Could you check a few things on this model? Use its own coordinates, in mm. Face numbers are marked on the shaded views. A direction names the side the tool comes from. Coordinates: 2 decimals unless noted, no trailing zeros. Loops run counter-clockwise (first coordinate to the right, second up) from the corner with the lowest first, then second, coordinate; pieces in that order, holes last. Notation, with made-up numbers: (-4, 42) - (54, 42) arc R14 cw to (54, 46) - close; hole circle Ø9 at (75, 46.5). An arc over 180 degrees is marked (long way). Use CSV: the item, a comma, the result in double quotes.
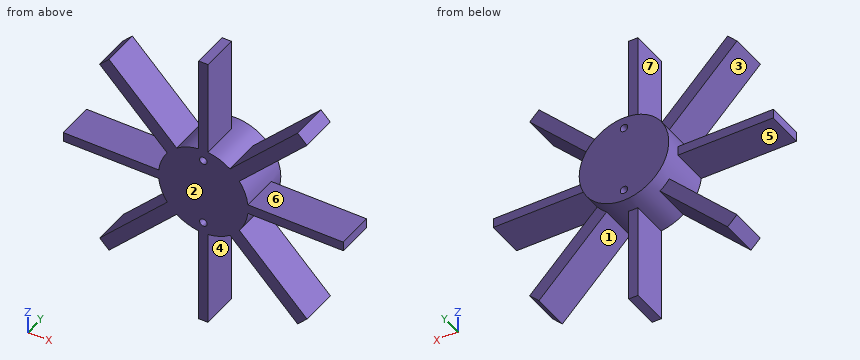
Autodesk Inventor part; units mm, degrees
ref_plane "YZ Plane" through (0, 0, 0) normal (1, 0, 0) x (0, 1, 0)
ref_plane "XZ Plane" through (0, 0, 0) normal (0, 1, 0) x (-1, 0, 0)
ref_plane "XY Plane" through (0, 0, 0) normal (0, 0, 1) x (1, 0, 0)
sketch "Sketch2" plane through (0, 0, 0) normal (0, 1, 0) x (-1, 0, 0)
  circle A0 centre (0, 0) radius 12
  line L0 (-1.25, 37.5) -> (-1.25, -37.5)
  line L1 (-1.25, -37.5) -> (1.25, -37.5)
  line L2 (1.25, -37.5) -> (1.25, 37.5)
  line L3 (1.25, 37.5) -> (-1.25, 37.5)
  line L4 (-1.25, 37.5) -> (1.25, -37.5) construction
  line L5 (-1.25, -37.5) -> (1.25, 37.5) construction
  line L6 (-37.5, -1.25) -> (37.5, -1.25)
  line L7 (37.5, -1.25) -> (37.5, 1.25)
  line L8 (37.5, 1.25) -> (-37.5, 1.25)
  line L9 (-37.5, 1.25) -> (-37.5, -1.25)
  line L10 (-37.5, -1.25) -> (37.5, 1.25) construction
  line L11 (37.5, -1.25) -> (-37.5, 1.25) construction
  line L12 (1.25, 1.25) -> (-1.25, -1.25)
  line L13 (-1.25, -1.25) -> (25.2665, -27.7665)
  line L14 (25.2665, -27.7665) -> (27.7665, -25.2665)
  line L15 (27.7665, -25.2665) -> (1.25, 1.25)
  line L16 (1.25, 1.25) -> (-1.25, -1.25)
  line L17 (-1.25, -1.25) -> (-27.7665, 25.2665)
  line L18 (-27.7665, 25.2665) -> (-25.2665, 27.7665)
  line L19 (-25.2665, 27.7665) -> (1.25, 1.25)
  line L20 (-1.25, 1.25) -> (1.25, -1.25)
  line L21 (1.25, -1.25) -> (-25.2665, -27.7665)
  line L22 (-25.2665, -27.7665) -> (-27.7665, -25.2665)
  line L23 (-27.7665, -25.2665) -> (-1.25, 1.25)
  line L24 (-1.25, 1.25) -> (1.25, -1.25)
  line L25 (1.25, -1.25) -> (27.7665, 25.2665)
  line L26 (27.7665, 25.2665) -> (25.2665, 27.7665)
  line L27 (25.2665, 27.7665) -> (-1.25, 1.25)
  point P0 (7.1427, -9.6427)
  point P1 (9.6427, -7.1427)
  point P2 (11.9347, -1.25)
  point P3 (11.9347, 1.25)
  point P4 (9.6427, 7.1427)
  point P5 (7.1427, 9.6427)
  point P6 (1.25, 11.9347)
  point P7 (-1.25, 11.9347)
  point P8 (-7.1427, 9.6427)
  point P9 (-9.6427, 7.1427)
  point P10 (-11.9347, 1.25)
  point P11 (-11.9347, -1.25)
  point P12 (-9.6427, -7.1427)
  point P13 (-7.1427, -9.6427)
  point P14 (-1.25, -11.9347)
  point P15 (1.25, -11.9347)
  dimension "d0" = 24
  dimension "d1" = 75
  dimension "d2" = 2.5
  dimension "d3" = 75
  dimension "d4" = 2.5
  dimension "d5" = 37.5
  dimension "d6" = 37.5
  dimension "d7" = 37.5
  dimension "d8" = 37.5
extrude "Extrusion1" add sketch "Sketch2" along normal blind 10
sketch "Sketch3" plane through (0, 10, 0) normal (0, 1, 0) x (1, 0, 0)
  circle A0 centre (0, 0) radius 12
  dimension "d11" = 24
extrude "Extrusion2" add sketch "Sketch3" along normal blind 4
sketch "Sketch4" plane through (0, 14, 0) normal (0, 1, 0) x (1, 0, 0)
  line L0 (0, 0) -> (0, 12)
  line L1 (1.25, 11.9347) -> (1.25, 37.5)
  line L2 (0, 0) -> (12, 0) construction
  line L3 (0, 12) -> (0, -12)
  line L4 (0, -12) -> (0, -9)
  line L5 (0, -12) -> (3, -12) construction
  line L6 (0, 12) -> (0, 9)
  line L7 (0, 12) -> (3, 12) construction
  circle A0 centre (0, -9) radius 1
  circle A1 centre (0, 9) radius 1
  dimension "d14" = 12
  dimension "d15" = 90
  dimension "d16" = 24
  dimension "d17" = 0
  dimension "d18" = 3
  dimension "d19" = 90
  dimension "d20" = 3
  dimension "d21" = 90
  dimension "d22" = 2
  dimension "d23" = 2
extrude "Extrusion3" cut sketch "Sketch4" against normal blind 20
properties part number "sweeper"
(1) Suppose I cut it at D-D (z = 0). Write out the boundary of the cut face in (x, y), plus the area to 3 significant figures.
Computed:
outline,"(-37.5, 0) - (37.5, 0) - (37.5, 10) - (12, 10) - (12, 14) - (-12, 14) - (-12, 10) - (-37.5, 10) - close"
area,"846 mm²"
(2) Thinking about a two-plate mould opening in X: for the marked faces 1, 2 and 3, which applies, +X half, -X half, draft (parallel to the pull), parting line (faces both ways), or undercut?
Computed:
face 1,"undercut"
face 2,"draft"
face 3,"-X half"
(3) Suppose I cut it at C-C (y = 2.75). State how many separate pieces and enclosed holes the cut face has, plus the area to 3 significant figures.
Computed:
separate pieces,"1"
enclosed holes,"2"
area,"1,060 mm²"
(4) Please list where these lines run through material, in increasing order: line 1 (Z direction, x = 0, y = 4.5); line 2 (Z direction, x = 17.5, y = 3); line 3 (X direction, y = 5.75, z = 20.5).
Computed:
line 1,"z = -37.5 to -10, -8 to 8, 10 to 37.5"
line 2,"z = -20 to -15, -1.25 to 1.25, 15 to 20"
line 3,"x = -23 to -18, -1.25 to 1.25, 18 to 23"
(5) Which directions (+Z, -Z, +X, -X, +Y, -Y) give clear straight access to the entire face, cutting with the end or side of a thin tool? Please do the marked faces 4, 5, 6 and 7.
Computed:
face 4,"-Z, +Y, -Y"
face 5,"-X, +Y, -Y"
face 6,"+X, +Y, -Y"
face 7,"+Z, +Y, -Y"
(6) Will these pins go through, and if not, where does the flat tip stop? pin 1 (22.5 mm diameter, centred on x = -21.5, z = -12.5, fed in from +Y); pin 2 (5 mm diameter, centred on x = -30.5, y = 3, fed in from -Z); pin 3 (5 mm diameter, centred on y = 7, z = -24, fed in from +X); pin 4 (5 mm diameter, centred on x = -14.5, z = -12, fed in from -Y).
Computed:
pin 1,"stops at y = 10"
pin 2,"stops at z = -1.25"
pin 3,"stops at x = 27.77"
pin 4,"stops at y = 0"
(7) Suppose I cut it at A-A (z = -21.5). Write out the boundary of the cut face in (x, y).
Computed:
outline,"(-24, 0) - (-19, 0) - (-19, 10) - (-24, 10) - close; (-1.25, 0) - (1.25, 0) - (1.25, 10) - (-1.25, 10) - close; (19, 0) - (24, 0) - (24, 10) - (19, 10) - close"
(8) Suppose I cut it at B-B (x = -18). Write out the boundary of the cut face in (y, z), plus the area to 3 significant figures.
Computed:
outline,"(0, -20.5) - (10, -20.5) - (10, -15.5) - (0, -15.5) - close; (0, -1.25) - (10, -1.25) - (10, 1.25) - (0, 1.25) - close; (0, 15.5) - (10, 15.5) - (10, 20.5) - (0, 20.5) - close"
area,"125 mm²"
